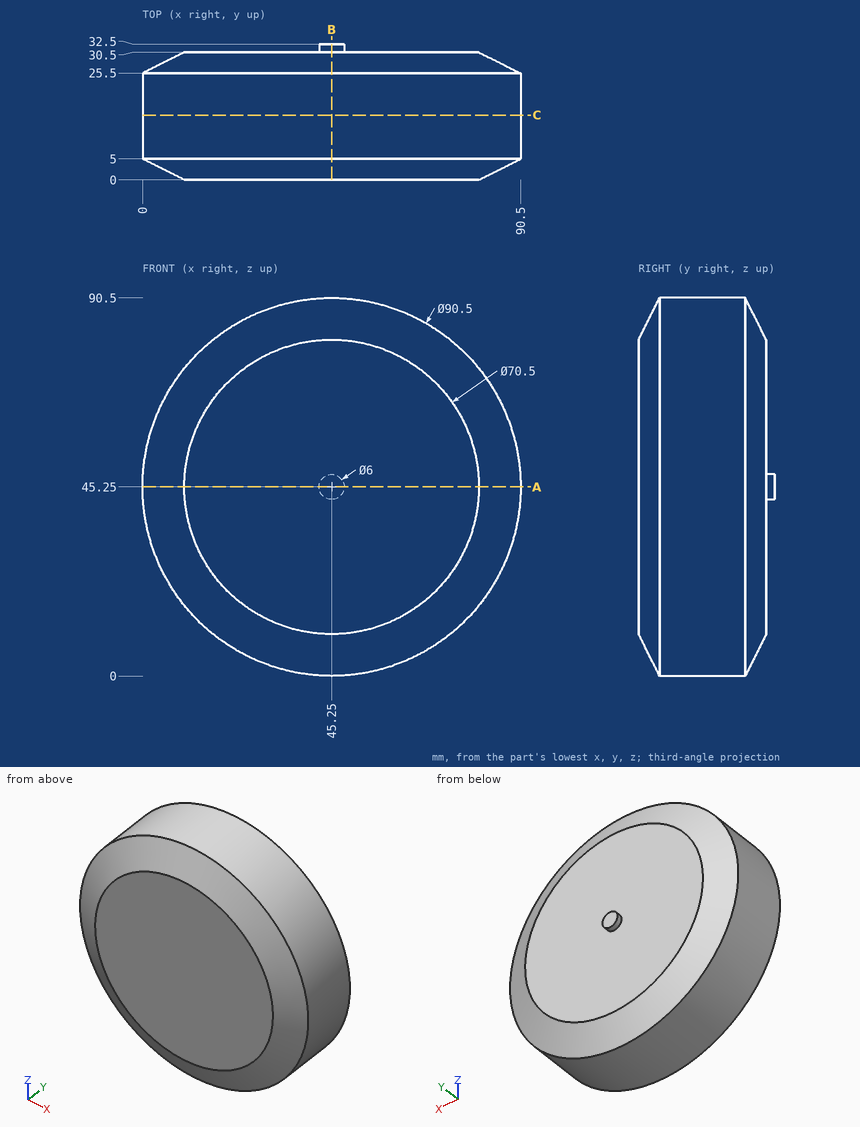
Source: three-view drawing plus pictorial views. Frame: mm from the lowest corner of the part. Give positions to 0.01 mm unless a question says otherwise; leave off trailing zeros. Write each loop counter-clockwise with the first axis right and the second up, starting at its lowest first coordinate (ties: lowest second). Pieces come first, ordered by that corner, then holes. Notation, with made-up numbers: (53.5, 11.25) -> (88.5, 11.25) arc R19 ccw to (88.5, 26.25) -> close; hole circle Ø11 at (9.25, 63.5). An arc over 180 degrees is marked (long way). Answer in a Markdown table with one row per item.
(1) Section query C-C on y = 15.5. Return loops of the section in (x, z), then the cut area to 3 significant figures.
Answers below:
| item | result |
|---|---|
| outline | circle Ø90.5 at (45.25, 45.25) |
| area | 6,430 mm^2 |
(2) Section query B-B on x = 45.25. Return loops of the section in (y, z), then the cut area to 3 significant figures.
Answers below:
| item | result |
|---|---|
| outline | (0, 10) -> (5, 0) -> (25.5, 0) -> (30.5, 10) -> (30.5, 42.25) -> (32.5, 42.25) -> (32.5, 48.25) -> (30.5, 48.25) -> (30.5, 80.5) -> (25.5, 90.5) -> (5, 90.5) -> (0, 80.5) -> close |
| area | 2,670 mm^2 |
(3) Ray query, line 1 along Y through (x, z) = (34, 22); line 2 along Z through (x, y) = (50.5, 9); line 3 along Z through (x, y) = (59.5, 24). Return the intervals inside material, ascending. Write a range as [from, to].
Answers below:
| item | result |
|---|---|
| line 1 | [0, 30.5] |
| line 2 | [0.31, 90.19] |
| line 3 | [2.3, 88.2] |
(4) Section query A-A on z = 45.25. Return loops of the section in (x, y).
Answers below:
| item | result |
|---|---|
| outline | (0, 5) -> (10, 0) -> (80.5, 0) -> (90.5, 5) -> (90.5, 25.5) -> (80.5, 30.5) -> (48.25, 30.5) -> (48.25, 32.5) -> (42.25, 32.5) -> (42.25, 30.5) -> (10, 30.5) -> (0, 25.5) -> close |
(5) Pin query (flat end, axial travel): pin 1 (2 mm diameter, centred on x = 40.5, z = 41, fed in from +Y); pin 2 (1.5 mm diameter, centred on y = 8.5, z = 14.5, fed in from -X); pin 3 (2 mm diameter, centred on x = 26, y = 7, fed in from +Z). Return the tip coordinate at first contact, or that it passes through.
Answers below:
| item | result |
|---|---|
| pin 1 | y = 30.5 |
| pin 2 | x = 11.37 |
| pin 3 | z = 86.66 |
